```python
from build123d import *

# Parameters (mm, degrees)
EXTRUDE_START                = -5
EXTRUDE_1_DEPTH              = 170
CUT_EXTRUDE_1_DEPTH          = 239.641991276
CUT_EXTRUDE_1_DEPTH_BACK     = 239.641991276
CUT_EXTRUDE_START            = -121.972243623
CUT_EXTRUDE_2_DEPTH          = 121.972243623
CUT_EXTRUDE_START_2          = -53.027756377
CUT_EXTRUDE_2_2_DEPTH        = 28.027756377
CUT_EXTRUDE_START_3          = -12.480754415
CUT_EXTRUDE_2_3_DEPTH        = 15
SKETCH_5_R                   = 55
EXTRUDE_2_DEPTH              = 60.5
SKETCH_6_W                   = 260
SKETCH_6_H                   = 200
EXTRUDE_3_DEPTH              = 25
CUT_EXTRUDE_3_DEPTH          = 5
FILLET_1_R                   = 12
SKETCH_9_R                   = 57.5
EXTRUDE_4_DEPTH              = 5
SKETCH_10_R                  = 50
EXTRUDE_5_DEPTH              = 30
CUT_EXTRUDE_4_DEPTH          = 332.888535558
CUT_EXTRUDE_4_DEPTH_BACK     = 332.888535558
SKETCH_11_R                  = 35
CUT_EXTRUDE_5_DEPTH          = 314.289004012
CUT_EXTRUDE_5_DEPTH_BACK     = 8
SKETCH_12_R                  = 26.5
CUT_EXTRUDE_6_REACH          = 309.594
SKETCH_13_R                  = 16
RIB_START                    = -7.5
RIB_1_DEPTH                  = 15
RIB_2_REACH                  = 278.451
SKETCH_15_WALL_W             = 586.29307431
SKETCH_15_WALL_H             = 15
HOLE_WIZARD_M6_1_D           = 5
HOLE_WIZARD_M6_1_DEPTH       = 22
HOLE_WIZARD_M6_1_CSINK_D     = 6.05
HOLE_WIZARD_M6_1_CSINK_ANGLE = 90
HOLE_WIZARD_M6_1_TIP         = 1.502151548
HOLE_WIZARD_M6_2_D           = 5
HOLE_WIZARD_M6_2_DEPTH       = 22
HOLE_WIZARD_M6_2_CSINK_D     = 6.05
HOLE_WIZARD_M6_2_CSINK_ANGLE = 90
HOLE_WIZARD_M6_2_TIP         = 1.502151548


with BuildPart() as part:
    # 草图1 → 凸台-拉伸1 (new body)
    with BuildSketch(Plane.XY.offset(EXTRUDE_START)):
        with BuildLine():
            Line((-90, 0), (-90, 135))
            Line((-90, 135), (90, 135))
            Line((90, 135), (90, 0))
            ThreePointArc((90, 0), (0, -90), (-90, 0))
        make_face()
    extrude(amount=-EXTRUDE_1_DEPTH)

    # 草图2 → 切除-拉伸1 (cut, two sides: drawn at the far end of the back side and taken through both)
    with BuildSketch(Plane(origin=(0, 0, 0), x_dir=(0, 0, -1), z_dir=(1, 0, 0)).offset(-CUT_EXTRUDE_1_DEPTH_BACK)):
        Polygon((338.831049921, -530.746574882), (45, -90), (5, -30), (-288.831049921, 410.746574882), (-1170.324199685, -176.915524961), (-542.662099843, -1118.408674725), align=None)
    extrude(amount=CUT_EXTRUDE_1_DEPTH + CUT_EXTRUDE_1_DEPTH_BACK, mode=Mode.SUBTRACT)

    # 切除-拉伸2: read off the stored shape, not the designer's step
    # 切除-拉伸2 outline → 切除-拉伸2 (cut)
    with BuildSketch(Plane(origin=(0, 0, -175), x_dir=(-1, 0, 0), z_dir=(0, 0, -1)).offset(CUT_EXTRUDE_START)):
        with BuildLine():
            Line((75, 115), (-75, 115))
            Line((-75, 115), (-75, 0))
            ThreePointArc((-75, 0), (0, -75), (75, 0))
            Line((75, 0), (75, 115))
        make_face()
    extrude(amount=CUT_EXTRUDE_2_DEPTH, mode=Mode.SUBTRACT)

    # Cut-Extrude 2 2 outline → Cut-Extrude 2 2 (cut)
    with BuildSketch(Plane.XY.offset(CUT_EXTRUDE_START_2)):
        with BuildLine():
            ThreePointArc((-75, 0), (0, -75), (75, 0))
            Line((75, 0), (75, 115))
            Line((75, 115), (-75, 115))
            Line((-75, 115), (-75, 0))
        make_face()
    extrude(amount=CUT_EXTRUDE_2_2_DEPTH, mode=Mode.SUBTRACT)

    # Cut-Extrude 2 3 outline → Cut-Extrude 2 3 (add)
    with BuildSketch(Plane(origin=(0, 0, 0), x_dir=(1, 0, 0), z_dir=(0, 0.5547001962252289, -0.8320502943378438)).offset(CUT_EXTRUDE_START_3)):
        with BuildLine():
            Line((-67.370217069, 41.290522566), (67.370217069, 41.290522566))
            add(Edge.make_bspline(
                [(67.370217069, 41.290522566), (0, 206.799154918), (-67.370217069, 41.290522566)],
                knots=[5.167369564, 5.167369564, 5.167369564, 7.399001051, 7.399001051, 7.399001051], degree=2, weights=[1, 0.439444872, 1]))
        make_face()
    extrude(amount=CUT_EXTRUDE_2_3_DEPTH)

    # 草图5 → 凸台-拉伸2 (add)
    with BuildSketch(Plane.XY):
        Circle(SKETCH_5_R)
    extrude(amount=-EXTRUDE_2_DEPTH)

    # 草图6 → 凸台-拉伸3 (add)
    with BuildSketch(Plane.XY):
        with Locations((0, 70)):
            Rectangle(SKETCH_6_W, SKETCH_6_H)
    extrude(amount=-EXTRUDE_3_DEPTH)

    # 草图8 → 切除-拉伸3 (cut)
    with BuildSketch(Plane.XY):
        with BuildLine():
            Line((-90, -30), (-90, 120))
            Line((-90, 120), (90, 120))
            Line((90, 120), (90, -30))
            Line((90, -30), (46.097722286, -30))
            ThreePointArc((46.097722286, -30), (0, 55), (-46.097722286, -30))
            Line((-46.097722286, -30), (-90, -30))
        make_face()
    extrude(amount=-CUT_EXTRUDE_3_DEPTH, mode=Mode.SUBTRACT)

    # 圆角1
    fillet_1_edges = [part.edges().sort_by_distance(p)[0] for p in [
        (130, -30, -12.5),
        (130, 170, -12.5),
        (-130, -30, -12.5),
        (-130, 170, -12.5),
    ]]
    fillet(fillet_1_edges, radius=FILLET_1_R)

    # 草图9 → 凸台-拉伸4 (add)
    with BuildSketch(Plane(origin=(90, 0, 0), x_dir=(0, 0, -1), z_dir=(1, 0, 0))):
        with Locations(Location((107, 75, 0), (0, 0, 90))):
            Circle(SKETCH_9_R)
    extrude_4 = extrude(amount=EXTRUDE_4_DEPTH)

    # 草图10 → 凸台-拉伸5 (add)
    with BuildSketch(Plane.ZY.offset(-95)):
        with Locations((-107, 75)):
            Circle(SKETCH_10_R)
    extrude_5 = extrude(amount=EXTRUDE_5_DEPTH)

    # 镜向1: 凸台-拉伸4, 凸台-拉伸5 across plane
    add(extrude_4.mirror(Plane(origin=(0, 0, 0), x_dir=(0, 0, 1), z_dir=(1, 0, 0))))
    add(extrude_5.mirror(Plane(origin=(0, 0, 0), x_dir=(0, 0, 1), z_dir=(1, 0, 0))))

    # 草图11 → 切除-拉伸4 (cut, two sides: drawn at the far end of the back side and taken through both)
    with BuildSketch(Plane(origin=(95, 0, 0), x_dir=(0, 0, -1), z_dir=(1, 0, 0)).offset(-CUT_EXTRUDE_4_DEPTH_BACK)):
        with Locations(Location((107, 75, 0), (0, 0, 90))):
            Circle(SKETCH_11_R)
    extrude(amount=CUT_EXTRUDE_4_DEPTH + CUT_EXTRUDE_4_DEPTH_BACK, mode=Mode.SUBTRACT)

    # 草图12 → 切除-拉伸5 (cut, two sides: drawn at the far end of the back side and taken through both)
    with BuildSketch(Plane(origin=(0, 135, 0), x_dir=(1, 0, 0), z_dir=(0, 1, 0)).offset(-CUT_EXTRUDE_5_DEPTH_BACK)):
        with Locations((0, 87)):
            Circle(SKETCH_12_R)
    extrude(amount=CUT_EXTRUDE_5_DEPTH + CUT_EXTRUDE_5_DEPTH_BACK, mode=Mode.SUBTRACT)

    # 草图13 → 切除-拉伸6 (cut, up to next)
    with BuildSketch(Plane(origin=(0, 127, 0), x_dir=(1, 0, 0), z_dir=(0, 1, 0)), mode=Mode.PRIVATE) as cut_extrude_6_sk1:
        with Locations(Location((0, 87, 0), (0, 0, 180))):
            Circle(SKETCH_13_R)
    cut_extrude_6_tool1 = extrude(cut_extrude_6_sk1.sketch, amount=-CUT_EXTRUDE_6_REACH, mode=Mode.PRIVATE) & part.part
    add(cut_extrude_6_tool1.solids().sort_by_distance((0, 127, -87))[0], mode=Mode.SUBTRACT)

    # 筋1: read off the stored shape, not the designer's step
    # 筋1 outline → 筋1 (add)
    with BuildSketch(Plane(origin=(0, 0, 0), x_dir=(0, 0, -1), z_dir=(1, 0, 0)).offset(RIB_START)):
        Polygon((55.5, -76), (55.5, -53), (38.361089711, -53), (53.027756377, -75), (53.694423044, -76), align=None)
    extrude(amount=RIB_1_DEPTH)

    # 草图15 wall → 筋2 (add, up to next)
    with BuildSketch(Plane(origin=(59.304181844, 0, -55.5), x_dir=(-1, 0, 0), z_dir=(0, 0, 1)), mode=Mode.PRIVATE) as rib_2_sk1:
        Rectangle(SKETCH_15_WALL_W, SKETCH_15_WALL_H)
    rib_2_tool1 = extrude(rib_2_sk1.sketch, amount=RIB_2_REACH, mode=Mode.PRIVATE) - part.part
    rib_2 = rib_2_tool1.solids().sort_by_distance((59.304181844, 0, -55.5))[0]
    add(rib_2)

    # 镜向4: 筋2 across plane
    add(rib_2.mirror(Plane(origin=(0, 0, 0), x_dir=(0, 0, 1), z_dir=(1, 0, 0))))

    # M6 螺纹孔1
    with Locations(Plane(origin=(0, 0, -175), x_dir=(-1, 0, 0), z_dir=(0, 0, -1))):
        with Locations((82, 125), (-82, 125)):
            CounterSinkHole(HOLE_WIZARD_M6_1_D / 2, HOLE_WIZARD_M6_1_CSINK_D / 2, depth=HOLE_WIZARD_M6_1_DEPTH, counter_sink_angle=HOLE_WIZARD_M6_1_CSINK_ANGLE)
            with Locations((0, 0, -(HOLE_WIZARD_M6_1_DEPTH + HOLE_WIZARD_M6_1_TIP / 2))):  # 118° drill point
                Cone(0, HOLE_WIZARD_M6_1_D / 2, HOLE_WIZARD_M6_1_TIP, mode=Mode.SUBTRACT)

    # M6 螺纹孔2
    with Locations(Plane(origin=(0, 0, -175), x_dir=(-1, 0, 0), z_dir=(0, 0, -1))):
        with Locations((0, -82)):
            CounterSinkHole(HOLE_WIZARD_M6_2_D / 2, HOLE_WIZARD_M6_2_CSINK_D / 2, depth=HOLE_WIZARD_M6_2_DEPTH, counter_sink_angle=HOLE_WIZARD_M6_2_CSINK_ANGLE)
            with Locations((0, 0, -(HOLE_WIZARD_M6_2_DEPTH + HOLE_WIZARD_M6_2_TIP / 2))):  # 118° drill point
                Cone(0, HOLE_WIZARD_M6_2_D / 2, HOLE_WIZARD_M6_2_TIP, mode=Mode.SUBTRACT)


solid = part.part
```
Check sheet for the modelled part. Datum: model origin and axes. Units: mm. A direction names the side the tool comes from. Round coordinates to 2 decimals unless told otherwise and drop trailing zeros. Order: outer loops, then holes, each group sorted by start corner. A loop starts at its lowest first (then second) coordinate and runs counter-clockwise, first axis right, second up. Notation, with made-up numbers: (-21.75, 5.25) -> (30.25, 5.25) arc R11 ccw to (30.25, 17.25) -> close; hole circle Ø3 at (-21.75, 39). An arc over 180 degrees is marked (long way). One line per item, written item: value. Start each with the question number.
Q1. Cross-section at C-C (x = 107.5). Record the boundary of the cut face in (y, z), and give its area (3 significant figures).
Q2. Gauge pin test, flat ends, axial feed: pin 1 Ø16.5 at (x, y) = (-69.5, -2.5) entering from -Z; pin 2 Ø1 at (x, z) = (-8, -43) entering from -Y; pin 3 Ø4.5 at (x, y) = (0, -82) entering from -Z; pin 4 Ø1.5 at (x, z) = (39, -74) entering from +Y. Record the tip position at first contact, or that the pin passes through.
Q3. Mould release check, pull along X, two halves, no side actions. Record for faces 6 (the face through (-95, 50, -82)), 7 (the face through (0, -65, -55.5)), 8 (the face through (-1, -60, -25)): pulls with the +X half, pulls with the -X half, needs draft (parallel to the pull), parting line crosses it, or undercut.
Q4. Thickness scan on line 1 (X direction, y = 125, z = -167.75); line 2 (Y direction, x = 0, z = -167); line 3 (Z direction, x = 89, y = 75). Record the ranges inside material, lowest first.
Q5. Cross-section at B-B (y = -13). Record the boundary of the cut face in (x, z).
Q6. Cross-section at D-D (z = -14). Record the boundary of the cut face in (x, y).
Q7. Set-up check for faces 1 (the face through (29.568, 46.376, -42.501)), 2 (the face through (130, 69, -12)), 3 (the face through (2.083, 121.084, -71.136)), 4 (the face through (-92.465, 62.535, -163.133)), 5 (the face through (-75, 31, -82)): record each of +Z, -Z, +X, -X, +Y, -Y from which the full face is reachable in a straight line by a thin tool's end or side.
Q8. Cross-section at A-A (z = -148). Record the boundary of the cut face in (x, y).
Completed:
1. outline: (-30, -25) -> (170, -25) -> (170, 0) -> (-30, 0) -> close
1. area: 5,000 mm²
2. pin 1: stops at z = -175
2. pin 2: stops at y = -87.75
2. pin 3: stops at z = -152.85
2. pin 4: stops at y = 135
3. face 6: pulls with the -X half
3. face 7: undercut
3. face 8: needs draft
4. line 1: x = -90 to -84.5, -79.5 to 79.5, 84.5 to 90
4. line 2: y = -90 to -84.5, -79.5 to -75, 115 to 135
4. line 3: z = -175 to -142, -72 to -5
5. outline: (-130, -25) -> (-89.06, -25) -> (-89.06, -175) -> (-73.86, -175) -> (-73.86, -25) -> (-53.44, -25) -> (-53.44, -60.5) -> (53.44, -60.5) -> (53.44, -25) -> (73.86, -25) -> (73.86, -175) -> (89.06, -175) -> (89.06, -25) -> (130, -25) -> (130, 0) -> (90, 0) -> (90, -5) -> (53.44, -5) -> (53.44, 0) -> (-53.44, 0) -> (-53.44, -5) -> (-90, -5) -> (-90, 0) -> (-130, 0) -> close
6. outline: (-130, -18) arc R12 ccw to (-118, -30) -> (-84.85, -30) arc R90 ccw to (-78.79, -43.5) -> (-33.66, -43.5) arc R55 ccw to (33.66, -43.5) -> (78.79, -43.5) arc R90 ccw to (84.85, -30) -> (118, -30) arc R12 ccw to (130, -18) -> (130, 158) arc R12 ccw to (118, 170) -> (-118, 170) arc R12 ccw to (-130, 158) -> close
7. face 1: -Z
7. face 2: +Z, -Z, +X, +Y, -Y
7. face 3: +Y
7. face 4: -X
7. face 5: none
8. outline: (-95, 34.69) -> (-90, 34.69) -> (-90, 0) arc R90 ccw to (90, 0) -> (90, 34.69) -> (95, 34.69) -> (95, 115.31) -> (90, 115.31) -> (90, 135) -> (-90, 135) -> (-90, 115.31) -> (-95, 115.31) -> close; hole (-75, 0) arc R75 ccw to (75, 0) -> (75, 46.38) -> (65, 46.38) -> (65, 103.62) -> (75, 103.62) -> (75, 115) -> (-75, 115) -> (-75, 103.62) -> (-65, 103.62) -> (-65, 46.38) -> (-75, 46.38) -> close
